from build123d import *

# Parameters (mm, degrees)
BOSS_EXTRUDE1_DEPTH = 3
SKETCH4_W           = 4.5
SKETCH4_H           = 5
BOSS_EXTRUDE3_DEPTH = 12
SKETCH5_W           = 5
SKETCH5_H           = 4
BOSS_EXTRUDE4_DEPTH = 12
SKETCH6_R           = 1.5
CUT_EXTRUDE1_DEPTH  = 10
SKETCH7_R           = 1.5
CUT_EXTRUDE2_DEPTH  = 10
SKETCH8_W           = 23
SKETCH8_H           = 2
BOSS_EXTRUDE5_DEPTH = 8
SKETCH11_W          = 23
SKETCH11_H          = 8
BOSS_EXTRUDE7_DEPTH = 3.5
SKETCH12_W          = 2
SKETCH12_H          = 5
CUT_EXTRUDE3_DEPTH  = 27.5
FILLET1_R           = 2
SKETCH13_W          = 4
SKETCH13_H          = 12
BOSS_EXTRUDE8_DEPTH = 3.5
SKETCH14_W          = 2
SKETCH14_H          = 9
CUT_EXTRUDE4_DEPTH  = 10
FILLET2_R           = 2


with BuildPart() as part:
    # Sketch1 → Boss-Extrude1 (new body)
    with BuildSketch(Plane(origin=(0, 0, 0), x_dir=(1, 0, 0), z_dir=(0, 1, 0))):
        Polygon((-14.802642583, 11.589093702), (-14.802642583, -10.410906298), (8.197357417, -10.410906298), (8.197357417, 11.589093702), (13.197357417, 11.589093702), (13.197357417, 15.589093702), (8.197357417, 15.589093702), (8.197357417, 22.589093702), (-14.802642583, 22.589093702), (-14.802642583, 15.589093702), (-19.802642583, 15.589093702), (-19.802642583, 11.589093702), align=None)
    extrude(amount=BOSS_EXTRUDE1_DEPTH)

    # Sketch4 → Boss-Extrude3 (add)
    with BuildSketch(Plane.XZ):
        with Locations((5.947357417, -20.089093702)):
            Rectangle(SKETCH4_W, SKETCH4_H)
        with Locations((5.947357417, 7.910906298)):
            Rectangle(SKETCH4_W, SKETCH4_H)
    extrude(amount=BOSS_EXTRUDE3_DEPTH)

    # Sketch5 → Boss-Extrude4 (add)
    with BuildSketch(Plane(origin=(0, 3, 0), x_dir=(1, 0, 0), z_dir=(0, 1, 0))):
        with Locations((-17.302642583, 13.589093702)):
            Rectangle(SKETCH5_W, SKETCH5_H)
        with Locations((10.697357417, 13.589093702)):
            Rectangle(SKETCH5_W, SKETCH5_H)
    extrude(amount=BOSS_EXTRUDE4_DEPTH)

    # Sketch6 → Cut-Extrude1 (cut)
    with BuildSketch(Plane.XY.offset(-11.589093702)):
        with Locations((-17.302642583, 9)):
            Circle(SKETCH6_R)
        with Locations((10.697357417, 9)):
            Circle(SKETCH6_R)
    extrude(amount=-CUT_EXTRUDE1_DEPTH, mode=Mode.SUBTRACT)

    # Sketch7 → Cut-Extrude2 (cut)
    with BuildSketch(Plane(origin=(8.197357417, 0, 0), x_dir=(0, 0, -1), z_dir=(1, 0, 0))):
        with Locations((-7.910906298, -6)):
            Circle(SKETCH7_R)
        with Locations((20.089093702, -6)):
            Circle(SKETCH7_R)
    extrude(amount=-CUT_EXTRUDE2_DEPTH, mode=Mode.SUBTRACT)

    # Sketch8 → Boss-Extrude5 (add)
    with BuildSketch(Plane(origin=(0, 3, 0), x_dir=(1, 0, 0), z_dir=(0, 1, 0))):
        with Locations((-3.302642583, -9.410906298)):
            Rectangle(SKETCH8_W, SKETCH8_H)
    extrude(amount=BOSS_EXTRUDE5_DEPTH)

    # Sketch11 → Boss-Extrude7 (add)
    with BuildSketch(Plane.XY.offset(10.410906298)):
        with Locations((-3.302642583, 7)):
            Rectangle(SKETCH11_W, SKETCH11_H)
    extrude(amount=BOSS_EXTRUDE7_DEPTH)

    # Sketch12 → Cut-Extrude3 (cut)
    with BuildSketch(Plane.ZY.offset(14.802642583)):
        with Locations((11.410906298, 7)):
            Rectangle(SKETCH12_W, SKETCH12_H)
    extrude(amount=-CUT_EXTRUDE3_DEPTH, mode=Mode.SUBTRACT)

    # Fillet1
    fillet1_edges = [part.edges().sort_by_distance(p)[0] for p in [
        (-3.302642583, 3, 13.910906298),
        (-3.302642583, 11, 13.910906298),
    ]]
    fillet(fillet1_edges, radius=FILLET1_R)

    # Sketch13 → Boss-Extrude8 (add)
    with BuildSketch(Plane.ZY.offset(19.802642583)):
        with Locations((-13.589093702, 9)):
            Rectangle(SKETCH13_W, SKETCH13_H)
    extrude(amount=BOSS_EXTRUDE8_DEPTH)

    # Sketch14 → Cut-Extrude4 (cut)
    with BuildSketch(Plane.XY.offset(-11.589093702)):
        with Locations((-20.802642583, 9)):
            Rectangle(SKETCH14_W, SKETCH14_H)
    extrude(amount=-CUT_EXTRUDE4_DEPTH, mode=Mode.SUBTRACT)

    # Fillet2
    fillet2_edges = [part.edges().sort_by_distance(p)[0] for p in [
        (-23.302642583, 3, -13.589093702),
        (-23.302642583, 15, -13.589093702),
    ]]
    fillet(fillet2_edges, radius=FILLET2_R)


solid = part.part
CAD build for the part. Positions are in the model's coordinates, mm. A direction names the side the tool comes from. Round coordinates to 2 decimals unless told otherwise and drop trailing zeros. Write each loop counter-clockwise with the first axis right and the second up, starting at its lowest first coordinate (ties: lowest second). Pieces come first, ordered by that corner, then holes. Notation, with made-up numbers: M -3,31 L 43,31 A21 cw 43,68 Z; hole C 80,68 d11. An arc over 180 degrees is marked long. Use a Markdown table: item, result. Add a question column.
1. Slice it at C-C on x = -3. Give the cut face in (y, z), then the cut area to 3 significant figures.
2. Flat gauge pins, fed straight in: P1, Ø3.5, axis at y = -6, z = -18.5, coming from the +X side; P2, Ø10, axis at x = -4.5, y = 10.5, coming from the -Z side; P3, Ø1.3, axis at x = 5, y = -5, coming from the +Z side; P4, Ø6, axis at y = -3.5, z = -5.5, coming from the +X side (3 decimals). Where does each tip first touch, or does it go through?
3. 3-axis set-ups, long thin cutter, end or side, ignore diameter. For faces 4 (the face through (-19, 7, -11.589)), 5 (the face through (11, 7, -15.589)), 6 (the face through (8.197, 9, -14)), 7 (the face through (-19.803, 9, -14)), 8 (the face through (-21, 3, -14)): which of +Z, -Z, +X, -X, +Y, -Y reach the whole face in a straight line?
4. Slice it at A-A on y = 6. Give the cut face in (x, z), then the cut area to 4 significant figures.
5. Pull direction Z, two halves, no side cores. Call faces 1 (the face through (-3.14, 10.4, 13.34)), 2 (the face through (-3, 3, 11)), 3 (the face through (-3, 7, 12.411)): released by +Z, released by -Z, zero draft, split by the parting line, or undercut.
6. Drill centre lines: probe 1 along Z at (x, y) = (-6, 5.5); probe 2 along Y at (x, z) = (0.5, -5); probe 3 along Y at (x, z) = (-15, -14.5). Where is each one in solid material? Low to high.
7. Slice it at B-B on x = 6. Give the cut face in (y, z).
8. Slice it at D-D on y = -8. Give the cut face in (x, z).
Reply:
| question | item | result |
|---|---|---|
| 1 | outline | M 0,-22.59 L 3,-22.59 L 3,8.41 L 11,8.41 L 11,11.91 A2 ccw 9,13.91 L 5,13.91 A2 ccw 3,11.91 L 3,10.41 L 0,10.41 Z; hole M 4.5,10.41 L 9.5,10.41 L 9.5,12.41 L 4.5,12.41 Z |
| 1 | area | 131 mm^2 |
| 2 | P1 | stops at x = 8.2 |
| 2 | P2 | stops at z = 8.41 |
| 2 | P3 | stops at z = 10.41 |
| 2 | P4 | passes through |
| 3 | face 4 | +Z, -X, +Y, -Y |
| 3 | face 5 | -Z, +X, +Y, -Y |
| 3 | face 6 | -Z, +Y |
| 3 | face 7 | +Z, -Z |
| 3 | face 8 | +Z, -Z, -X, -Y |
| 4 | outline | M -23.3,-15.59 L -21.8,-15.59 L -21.8,-11.59 L -23.3,-11.59 Z; M -19.8,-15.59 L -14.8,-15.59 L -14.8,-11.59 L -19.8,-11.59 Z; M -14.8,8.41 L 8.2,8.41 L 8.2,10.41 L -14.8,10.41 Z; M -14.8,12.41 L 8.2,12.41 L 8.2,13.91 L -14.8,13.91 Z; M 8.2,-15.59 L 13.2,-15.59 L 13.2,-11.59 L 8.2,-11.59 Z |
| 4 | area | 126.5 mm^2 |
| 5 | face 1 | released by +Z |
| 5 | face 2 | zero draft |
| 5 | face 3 | undercut |
| 6 | probe 1 | z = 8.41 to 10.41, 12.41 to 13.91 |
| 6 | probe 2 | y = 0 to 3 |
| 6 | probe 3 | y = 0 to 15 |
| 7 | outline | M -12,-22.59 L 3,-22.59 L 3,8.41 L 11,8.41 L 11,11.91 A2 ccw 9,13.91 L 5,13.91 A2 ccw 3,11.91 L 3,10.41 L -12,10.41 L -12,5.41 L 0,5.41 L 0,-17.59 L -12,-17.59 Z; hole C -6,-20.09 d3; hole C -6,7.91 d3; hole M 4.5,10.41 L 9.5,10.41 L 9.5,12.41 L 4.5,12.41 Z |
| 8 | outline | M 3.7,-22.59 L 8.2,-22.59 L 8.2,-17.59 L 3.7,-17.59 Z; M 3.7,5.41 L 8.2,5.41 L 8.2,10.41 L 3.7,10.41 Z |
